The listing builds one solid part. Answer for the finished solid, in the listing's coordinates (mm). Round coordinates to 2 decimals unless told otherwise and drop trailing zeros. Order: outer loops, then holes, each group sorted by start corner. A loop starts at its lowest first (then second) coordinate and runs counter-clockwise, first axis right, second up. Notation, with made-up numbers: (-30.5, -23.75) - (-25.5, -23.75) arc R24 ccw to (-25.5, 3.25) - close; hole circle Ø10 at (-14, -3). An arc over 180 degrees is marked (long way). Use CSV: the item, a comma, the result in double quotes. Start each with the question number.
Item 1: Flat-ended cylindrical pins translate along their axes: P1, Ø1.5, axis at x = 195, z = 79.5, coming from the -Y side; P2, Ø8, axis at x = 191, z = 63, coming from the -Y side; P3, Ø2.5, axis at y = 197, z = 3.5, coming from the +X side; P4, Ø12, axis at x = 186.5, y = 179, coming from the +Z side. Find the tip coordinate at first contact, or state that the pin passes through.
Item 2: Straight lines are drawn through the part: line 1 along X through (y, z) = (172, 100.5); line 2 along Y through (x, z) = (193.75, 84); line 3 along X through (y, z) = (187.5, 163.5). For each, find the intervals that lie inside material, in ascending order. Write a range as [from, to].
Item 3: Find section A-A, the plane z = 147. Give the vertices of the cut face in (x, y), plus the area to 3 significant figures.
Item 4: Find section B-B, the plane x = 191.75. Give the vertices of the cut face in (y, z).
```python
from build123d import *

# Parameters (mm, degrees)
BOSS_EXTRUDE1_DEPTH     = 5
BOSS_EXTRUDE2_DEPTH     = 180
SKETCH3_R               = 1.25
CUT_EXTRUDE1_DEPTH      = 180
CUT_EXTRUDE1_DEPTH_BACK = 180


with BuildPart() as part:
    # Sketch1 → Boss-Extrude1 (new body)
    with BuildSketch(Plane.XY):
        with BuildLine():
            Line((176.569505492, 187.840095713), (176.899877953, 168.242969935))
            ThreePointArc((176.899877953, 168.242969935), (177.048290864, 167.735381874), (177.434829134, 167.374466097))
            Line((177.434829134, 167.374466097), (186.718316852, 162.499660601))
            ThreePointArc((186.718316852, 162.499660601), (187.200079416, 162.385162323), (187.67770885, 162.515834233))
            Line((187.67770885, 162.515834233), (196.791607056, 167.700786723))
            ThreePointArc((196.791607056, 167.700786723), (197.16576035, 168.074526398), (197.296979738, 168.586828559))
            Line((197.296979738, 168.586828559), (197.234516514, 172.292039484))
            ThreePointArc((197.234516514, 172.292039484), (197.304175726, 172.675951622), (197.515449261, 173.003982761))
            Line((197.515449261, 173.003982761), (200.266782587, 175.849671866))
            ThreePointArc((200.266782587, 175.849671866), (200.474929456, 176.169876136), (200.547857403, 176.544759328))
            Line((200.547857403, 176.544759328), (200.547857403, 179.779238985))
            ThreePointArc((200.547857403, 179.779238985), (200.468478786, 180.169695473), (200.242944865, 180.498164169))
            Line((200.242944865, 180.498164169), (197.341824739, 183.303090564))
            ThreePointArc((197.341824739, 183.303090564), (197.119614365, 183.623813941), (197.037054271, 184.005159933))
            Line((197.037054271, 184.005159933), (196.992324343, 186.658462241))
            ThreePointArc((196.992324343, 186.658462241), (197.009048268, 186.858204702), (197.065271311, 187.050599374))
            Line((197.065271311, 187.050599374), (200.096416454, 194.537254131))
            ThreePointArc((200.096416454, 194.537254131), (200.151063173, 194.721369242), (200.169505492, 194.912535449))
            Line((200.169505492, 194.912535449), (200.169505492, 201.285162323))
            ThreePointArc((200.169505492, 201.285162323), (200.023058882, 201.638715714), (199.669505492, 201.785162323))
            Line((199.669505492, 201.785162323), (198.569505492, 201.785162323))
            ThreePointArc((198.569505492, 201.785162323), (198.215952101, 201.638715714), (198.069505492, 201.285162323))
            Line((198.069505492, 201.285162323), (198.069505492, 199.185162323))
            ThreePointArc((198.069505492, 199.185162323), (192.419505492, 193.535162323), (186.769505492, 199.185162323))
            Line((186.769505492, 199.185162323), (186.769505492, 201.285162323))
            ThreePointArc((186.769505492, 201.285162323), (186.623058882, 201.638715714), (186.269505492, 201.785162323))
            Line((186.269505492, 201.785162323), (182.669505492, 201.785162323))
            ThreePointArc((182.669505492, 201.785162323), (182.315952101, 201.638715714), (182.169505492, 201.285162323))
            Line((182.169505492, 201.285162323), (182.169505492, 193.585162323))
            ThreePointArc((182.169505492, 193.585162323), (182.023058882, 193.231608933), (181.669505492, 193.085162323))
            Line((181.669505492, 193.085162323), (179.669505492, 193.085162323))
            ThreePointArc((179.669505492, 193.085162323), (179.315952101, 193.231608933), (179.169505492, 193.585162323))
            Line((179.169505492, 193.585162323), (179.169505492, 201.285162323))
            ThreePointArc((179.169505492, 201.285162323), (179.023058882, 201.638715714), (178.669505492, 201.785162323))
            Line((178.669505492, 201.785162323), (177.069505492, 201.785162323))
            ThreePointArc((177.069505492, 201.785162323), (176.715952101, 201.638715714), (176.569505492, 201.285162323))
            Line((176.569505492, 201.285162323), (176.569505492, 187.840095713))
        make_face()
        with BuildLine():
            Line((186.260276974, 189.669797845), (180.118302096, 186.175590732))
            ThreePointArc((180.118302096, 186.175590732), (179.744148802, 185.801851058), (179.612929414, 185.289548897))
            Line((179.612929414, 185.289548897), (179.869468758, 170.072076543))
            ThreePointArc((179.869468758, 170.072076543), (180.017881669, 169.564488482), (180.404419939, 169.203572705))
            Line((180.404419939, 169.203572705), (186.660683401, 165.918377698))
            ThreePointArc((186.660683401, 165.918377698), (187.142445966, 165.803879419), (187.6200754, 165.934551329))
            Line((187.6200754, 165.934551329), (193.762050278, 169.428758442))
            ThreePointArc((193.762050278, 169.428758442), (194.136203572, 169.802498117), (194.26742296, 170.314800278))
            Line((194.26742296, 170.314800278), (194.010883616, 185.532272632))
            ThreePointArc((194.010883616, 185.532272632), (193.862470704, 186.039860693), (193.475932435, 186.400776469))
            Line((193.475932435, 186.400776469), (187.219668972, 189.685971477))
            ThreePointArc((187.219668972, 189.685971477), (186.737906408, 189.800469755), (186.260276974, 189.669797845))
        make_face(mode=Mode.SUBTRACT)
    extrude(amount=BOSS_EXTRUDE1_DEPTH)

    # Sketch2 → Boss-Extrude2 (add)
    with BuildSketch(Plane.XY.offset(5)):
        with BuildLine():
            Line((185.765791725, 190.538983866), (179.623816847, 187.044776753))
            ThreePointArc((179.623816847, 187.044776753), (178.875510259, 186.297297404), (178.613071484, 185.272693082))
            Line((178.613071484, 185.272693082), (178.869610827, 170.055220728))
            ThreePointArc((178.869610827, 170.055220728), (179.16643665, 169.040044606), (179.93951319, 168.318213053))
            Line((179.93951319, 168.318213053), (186.195776652, 165.033018045))
            ThreePointArc((186.195776652, 165.033018045), (187.159301781, 164.804021489), (188.114560649, 165.065365309))
            Line((188.114560649, 165.065365309), (194.256535527, 168.559572421))
            ThreePointArc((194.256535527, 168.559572421), (195.004842115, 169.307051771), (195.26728089, 170.331656093))
            Line((195.26728089, 170.331656093), (195.010741546, 185.549128447))
            ThreePointArc((195.010741546, 185.549128447), (194.713915724, 186.564304569), (193.940839184, 187.286136122))
            Line((193.940839184, 187.286136122), (187.684575722, 190.57133113))
            ThreePointArc((187.684575722, 190.57133113), (186.721050593, 190.800327686), (185.765791725, 190.538983866))
        make_face()
        with BuildLine():
            Line((186.260276974, 189.669797845), (180.118302096, 186.175590732))
            ThreePointArc((180.118302096, 186.175590732), (179.744148802, 185.801851058), (179.612929414, 185.289548897))
            Line((179.612929414, 185.289548897), (179.869468758, 170.072076543))
            ThreePointArc((179.869468758, 170.072076543), (180.017881669, 169.564488482), (180.404419939, 169.203572705))
            Line((180.404419939, 169.203572705), (186.660683401, 165.918377698))
            ThreePointArc((186.660683401, 165.918377698), (187.142445966, 165.803879419), (187.6200754, 165.934551329))
            Line((187.6200754, 165.934551329), (193.762050278, 169.428758442))
            ThreePointArc((193.762050278, 169.428758442), (194.136203572, 169.802498117), (194.26742296, 170.314800278))
            Line((194.26742296, 170.314800278), (194.010883616, 185.532272632))
            ThreePointArc((194.010883616, 185.532272632), (193.862470704, 186.039860693), (193.475932435, 186.400776469))
            Line((193.475932435, 186.400776469), (187.219668972, 189.685971477))
            ThreePointArc((187.219668972, 189.685971477), (186.737906408, 189.800469755), (186.260276974, 189.669797845))
        make_face(mode=Mode.SUBTRACT)
    extrude(amount=BOSS_EXTRUDE2_DEPTH)

    # Sketch3 → Cut-Extrude1 (cut, two sides)
    with BuildSketch(Plane(origin=(181.684802759, 3.06288055, 0), x_dir=(0, 0, 1), z_dir=(-0.999857931, -0.016855815, 0))) as cut_extrude1_sk:
        with Locations((2.5, 195.771915061)):
            Circle(SKETCH3_R)
        Polygon((185, 187.503282827), (185, 161.625885339), (160, 161.625885339), align=None)
    extrude(amount=CUT_EXTRUDE1_DEPTH, mode=Mode.SUBTRACT)
    extrude(cut_extrude1_sk.sketch, amount=-CUT_EXTRUDE1_DEPTH_BACK, mode=Mode.SUBTRACT)


solid = part.part
```
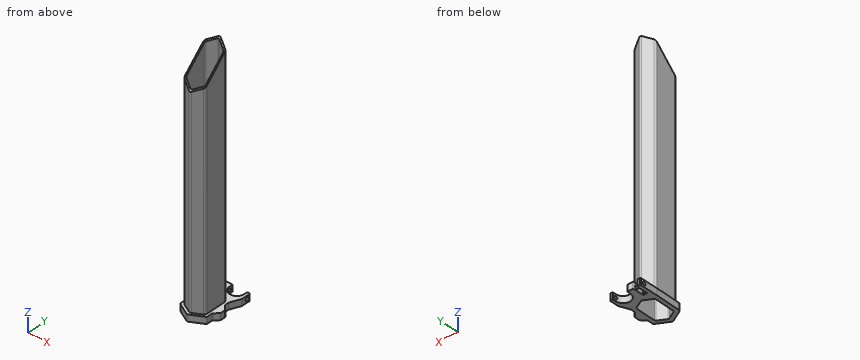
Worked out:
1,P1,"stops at y = 168.56"
1,P2,"stops at y = 164.8"
1,P3,"stops at x = 200.17"
1,P4,"passes through"
2,line 1,"x = [178.84, 179.84], [194.24, 195.24]"
2,line 2,"y = [168.27, 169.42], [186.19, 187.39]"
2,line 3,"x = [180.42, 182.45], [191.38, 193.53]"
3,outline,"(178.61, 185.27) - (178.87, 170.06) arc R2 ccw to (179.94, 168.32) - (186.2, 165.03) arc R2 ccw to (188.11, 165.07) - (194.26, 168.56) arc R2 ccw to (195.27, 170.33) - (195.01, 185.55) arc R2 ccw to (193.94, 187.29) - (187.68, 190.57) arc R2 ccw to (185.77, 190.54) - (179.62, 187.04) arc R2 ccw to start; hole (179.61, 185.29) - (179.87, 170.07) arc R1 ccw to (180.4, 169.2) - (186.66, 165.92) arc R1 ccw to (187.62, 165.93) - (193.76, 169.43) arc R1 ccw to (194.27, 170.31) - (194.01, 185.53) arc R1 ccw to (193.48, 186.4) - (187.22, 189.69) arc R1 ccw to (186.26, 189.67) - (180.12, 186.18) arc R1 ccw to start"
3,area,"68.1 mm²"
4,outline,"(164.83, 0) - (168.28, 0) - (168.28, 163.29) - (167.13, 162.18) - (167.13, 5) - (164.83, 5) - close; (187.31, 0) - (193.57, 0) - (193.57, 5) - (188.44, 5) - (188.44, 182.75) - (187.31, 181.66) - close"
